Can you work these out from the model? Positions are in its coordinate system, mm. Face numbers are marked on the shaded views. A direction names the side the tool comes from. Coordinates: 2 decimals unless noted, no trailing zeros. Loops run counter-clockwise (first coordinate to the right, second up) from the corner with the lowest first, then second, coordinate; pieces in that order, holes last.
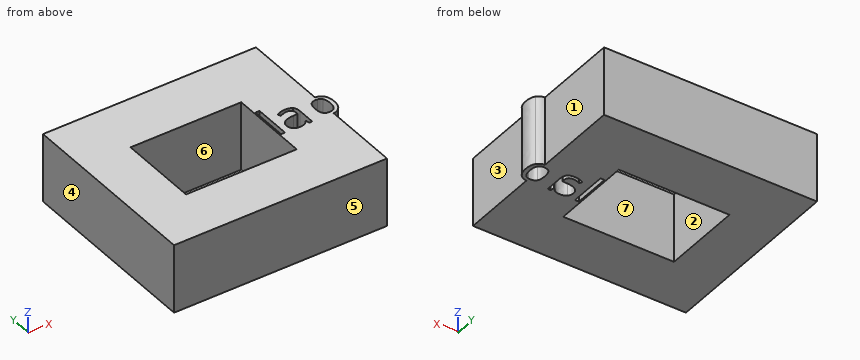
```python
from build123d import *

# Parameters (mm, degrees)
F0_W     = 1.4345356546
F0_H     = 13.4415161623
F1_DEPTH = 25


with BuildPart() as f1:
    # F0 (on Top) → F1 (new body)
    with BuildSketch(Plane.XY):
        Polygon((-19.7263322771, 14.6005926654), (-37.4334342778, 35.1035520434), (-37.4334342778, -33.8609479368), (-19.7263322771, -14.6005926654), align=None)
        Polygon((40.2292944491, 35.1035520434), (-37.4334342778, 35.1035520434), (-19.7263322771, 14.6005926654), (20.6582844257, 14.6005926654), align=None)
        with BuildLine():
            Line((40.2292944491, 4.0209012059), (40.2292944491, 35.1035520434))
            Line((40.2292944491, 35.1035520434), (20.6582844257, 14.6005926654))
            Line((20.6582844257, 14.6005926654), (20.6582844257, -14.6005926654))
            Line((20.6582844257, -14.6005926654), (40.2292944491, -33.8609479368))
            Line((40.2292944491, -33.8609479368), (40.2292944491, -5.7565652547))
            add(Edge.make_bspline(
                [(40.2292944491, -5.7565652547), (40.0783549242, -5.7658505375), (39.9216058908, -5.7658505375)],
                knots=[0.915231448, 0.915231448, 0.915231448, 1, 1, 1], degree=2))
            add(Edge.make_bspline(
                [(39.9216058908, -5.7658505375), (38.9956532043, -5.7658505375), (38.2313967333, -5.4244918605)],
                knots=[0, 0, 0, 1, 1, 1], degree=2))
            add(Edge.make_bspline(
                [(38.2313967333, -5.4244918605), (37.4671402622, -5.0831331836), (36.9502651805, -4.372775451)],
                knots=[0, 0, 0, 1, 1, 1], degree=2))
            Line((36.9502651805, -4.372775451), (36.8452317414, -4.372775451))
            Line((36.8452317414, -4.372775451), (36.5439516136, -5.5917161517))
            Line((36.5439516136, -5.5917161517), (35.5157295259, -5.5917161517))
            Line((35.5157295259, -5.5917161517), (35.5157295259, 7.8498000106))
            Line((35.5157295259, 7.8498000106), (36.9502651805, 7.8498000106))
            Line((36.9502651805, 7.8498000106), (36.9502651805, 4.5827072481))
            add(Edge.make_bspline(
                [(36.9502651805, 4.5827072481), (36.9502651805, 3.4853842137), (36.8811642337, 2.6147122846)],
                knots=[0, 0, 0, 1, 1, 1], degree=2))
            Line((36.8811642337, 2.6147122846), (36.9502651805, 2.6147122846))
            add(Edge.make_bspline(
                [(36.9502651805, 2.6147122846), (37.9508468894, 4.0298996741), (39.9216058908, 4.0298996741)],
                knots=[0, 0, 0, 1, 1, 1], degree=2))
            add(Edge.make_bspline(
                [(39.9216058908, 4.0298996741), (40.0783927276, 4.0298996741), (40.2292944491, 4.0209012059)],
                knots=[0, 0, 0, 0.0840353158, 0.0840353158, 0.0840353158], degree=2))
        make_face()
        with BuildLine():
            Line((32.5637370806, -5.5917161517), (31.4995825007, -5.5917161517))
            Line((31.4995825007, -5.5917161517), (31.2148866, -4.2428656711))
            Line((31.2148866, -4.2428656711), (31.1457856533, -4.2428656711))
            add(Edge.make_bspline(
                [(31.1457856533, -4.2428656711), (30.4381919585, -5.1328858652), (29.7347443206, -5.4493682014)],
                knots=[0, 0, 0, 1, 1, 1], degree=2))
            add(Edge.make_bspline(
                [(29.7347443206, -5.4493682014), (29.0312966827, -5.7658505375), (27.9754342163, -5.7658505375)],
                knots=[0, 0, 0, 1, 1, 1], degree=2))
            add(Edge.make_bspline(
                [(27.9754342163, -5.7658505375), (26.5685389404, -5.7658505375), (25.769731996, -5.0389085777)],
                knots=[0, 0, 0, 1, 1, 1], degree=2))
            add(Edge.make_bspline(
                [(25.769731996, -5.0389085777), (24.9709250515, -4.3119666178), (24.9709250515, -2.9741722887)],
                knots=[0, 0, 0, 1, 1, 1], degree=2))
            add(Edge.make_bspline(
                [(24.9709250515, -2.9741722887), (24.9709250515, -0.1078650174), (29.556463878, 0.0303368761)],
                knots=[0, 0, 0, 1, 1, 1], degree=2))
            Line((29.556463878, 0.0303368761), (31.1623698805, 0.0828535956))
            Line((31.1623698805, 0.0828535956), (31.1623698805, 0.6715936619))
            add(Edge.make_bspline(
                [(31.1623698805, 0.6715936619), (31.1623698805, 1.7855009236), (30.684191329, 2.3161961946)],
                knots=[0, 0, 0, 1, 1, 1], degree=2))
            add(Edge.make_bspline(
                [(30.684191329, 2.3161961946), (30.2060127774, 2.8468914657), (29.1501503111, 2.8468914657)],
                knots=[0, 0, 0, 1, 1, 1], degree=2))
            add(Edge.make_bspline(
                [(29.1501503111, 2.8468914657), (27.9671421027, 2.8468914657), (26.4745616528, 2.1227135437)],
                knots=[0, 0, 0, 1, 1, 1], degree=2))
            Line((26.4745616528, 2.1227135437), (26.0323155936, 3.2200365782))
            add(Edge.make_bspline(
                [(26.0323155936, 3.2200365782), (26.7316171747, 3.5987097664), (27.5649745926, 3.8143047202)],
                knots=[0, 0, 0, 1, 1, 1], degree=2))
            add(Edge.make_bspline(
                [(27.5649745926, 3.8143047202), (28.3983320104, 4.0298996741), (29.2385995229, 4.0298996741)],
                knots=[0, 0, 0, 1, 1, 1], degree=2))
            add(Edge.make_bspline(
                [(29.2385995229, 4.0298996741), (30.9301906994, 4.0298996741), (31.74696389, 3.2794633924)],
                knots=[0, 0, 0, 1, 1, 1], degree=2))
            add(Edge.make_bspline(
                [(31.74696389, 3.2794633924), (32.5637370806, 2.5290271106), (32.5637370806, 0.8706043886)],
                knots=[0, 0, 0, 1, 1, 1], degree=2))
            Line((32.5637370806, 0.8706043886), (32.5637370806, -5.5917161517))
        make_face(mode=Mode.SUBTRACT)
        with Locations((21.9208092619, 1.1290419294)):
            Rectangle(F0_W, F0_H, mode=Mode.SUBTRACT)
        Polygon((-19.7263322771, -14.6005926654), (-37.4334342778, -33.8609479368), (40.2292944491, -33.8609479368), (20.6582844257, -14.6005926654), align=None)
        with BuildLine():
            add(Edge.make_bspline(
                [(40.2292944491, 4.0209012059), (41.8740868362, 3.9228200715), (42.8196995976, 2.755678216)],
                knots=[0.0840353158, 0.0840353158, 0.0840353158, 1, 1, 1], degree=2))
            Line((40.2292944491, 4.0209012059), (40.2292944491, 2.7938202111))
            add(Edge.make_bspline(
                [(41.7168484874, 1.9237028171), (41.1987126844, 2.6484300811), (40.2292944491, 2.7938202111)],
                knots=[0, 0, 0, 0.7993864214, 0.7993864214, 0.7993864214], degree=2))
            add(Edge.make_bspline(
                [(42.365015368, -0.8320429394), (42.365015368, 1.0170983957), (41.7168484874, 1.9237028171)],
                knots=[0, 0, 0, 1, 1, 1], degree=2))
            add(Edge.make_bspline(
                [(41.7168484874, -3.6002268663), (42.365015368, -2.6369596686), (42.365015368, -0.8320429394)],
                knots=[0, 0, 0, 1, 1, 1], degree=2))
            add(Edge.make_bspline(
                [(40.2292944491, -4.528094354), (41.1929364436, -4.378833891), (41.7168484874, -3.6002268663)],
                knots=[0.1917019218, 0.1917019218, 0.1917019218, 1, 1, 1], degree=2))
            Line((40.2292944491, -4.528094354), (40.2292944491, -5.7565652547))
            add(Edge.make_bspline(
                [(42.811407484, -4.4736628332), (41.8589624891, -5.6563136569), (40.2292944491, -5.7565652547)],
                knots=[0, 0, 0, 0.915231448, 0.915231448, 0.915231448], degree=2))
            add(Edge.make_bspline(
                [(43.8520677421, -0.8486271666), (43.8520677421, -3.181475129), (42.811407484, -4.4736628332)],
                knots=[0, 0, 0, 1, 1, 1], degree=2))
            add(Edge.make_bspline(
                [(42.8196995976, 2.755678216), (43.8520677421, 1.4814567579), (43.8520677421, -0.8486271666)],
                knots=[0, 0, 0, 1, 1, 1], degree=2))
        make_face()
        with BuildLine():
            Line((40.2292944491, 2.7938202111), (40.2292944491, 4.0209012059))
            add(Edge.make_bspline(
                [(39.9216058908, 4.0298996741), (40.0783927276, 4.0298996741), (40.2292944491, 4.0209012059)],
                knots=[0, 0, 0, 0.0840353158, 0.0840353158, 0.0840353158], degree=2))
            add(Edge.make_bspline(
                [(36.9502651805, 2.6147122846), (37.9508468894, 4.0298996741), (39.9216058908, 4.0298996741)],
                knots=[0, 0, 0, 1, 1, 1], degree=2))
            Line((36.9502651805, 2.6147122846), (36.8811642337, 2.6147122846))
            add(Edge.make_bspline(
                [(36.9502651805, 4.5827072481), (36.9502651805, 3.4853842137), (36.8811642337, 2.6147122846)],
                knots=[0, 0, 0, 1, 1, 1], degree=2))
            Line((36.9502651805, 4.5827072481), (36.9502651805, 7.8498000106))
            Line((36.9502651805, 7.8498000106), (35.5157295259, 7.8498000106))
            Line((35.5157295259, 7.8498000106), (35.5157295259, -5.5917161517))
            Line((35.5157295259, -5.5917161517), (36.5439516136, -5.5917161517))
            Line((36.5439516136, -5.5917161517), (36.8452317414, -4.372775451))
            Line((36.8452317414, -4.372775451), (36.9502651805, -4.372775451))
            add(Edge.make_bspline(
                [(38.2313967333, -5.4244918605), (37.4671402622, -5.0831331836), (36.9502651805, -4.372775451)],
                knots=[0, 0, 0, 1, 1, 1], degree=2))
            add(Edge.make_bspline(
                [(39.9216058908, -5.7658505375), (38.9956532043, -5.7658505375), (38.2313967333, -5.4244918605)],
                knots=[0, 0, 0, 1, 1, 1], degree=2))
            add(Edge.make_bspline(
                [(40.2292944491, -5.7565652547), (40.0783549242, -5.7658505375), (39.9216058908, -5.7658505375)],
                knots=[0.915231448, 0.915231448, 0.915231448, 1, 1, 1], degree=2))
            Line((40.2292944491, -5.7565652547), (40.2292944491, -4.528094354))
            add(Edge.make_bspline(
                [(39.747471505, -4.563494064), (40.0007500207, -4.563494064), (40.2292944491, -4.528094354)],
                knots=[0, 0, 0, 0.1917019218, 0.1917019218, 0.1917019218], degree=2))
            add(Edge.make_bspline(
                [(37.6150162882, -3.7038782864), (38.279767396, -4.563494064), (39.747471505, -4.563494064)],
                knots=[0, 0, 0, 1, 1, 1], degree=2))
            add(Edge.make_bspline(
                [(36.9502651805, -0.8486271666), (36.9502651805, -2.8442625088), (37.6150162882, -3.7038782864)],
                knots=[0, 0, 0, 1, 1, 1], degree=2))
            add(Edge.make_bspline(
                [(37.598432061, 1.988657707), (36.9502651805, 1.1470081756), (36.9502651805, -0.8486271666)],
                knots=[0, 0, 0, 1, 1, 1], degree=2))
            add(Edge.make_bspline(
                [(39.7143030506, 2.8303072385), (38.2465989415, 2.8303072385), (37.598432061, 1.988657707)],
                knots=[0, 0, 0, 1, 1, 1], degree=2))
            add(Edge.make_bspline(
                [(40.2292944491, 2.7938202111), (39.9860097796, 2.8303072385), (39.7143030506, 2.8303072385)],
                knots=[0.7993864214, 0.7993864214, 0.7993864214, 1, 1, 1], degree=2))
        make_face()
    extrude(amount=F1_DEPTH)


solid = f1.part
```
(1) I want a section at C-C on z = 8.25. State how many separate pieces and enclosed holes the cut face has, then the cut area to 3 significant figures.
Check values:
separate pieces: 1
enclosed holes: 4
area: 4,100 mm2
(2) I want a section at B-B on y = -10.5. Write out the boundary of the cut face in (x, z).
Check values:
outline: (-37.43, 0) - (-19.73, 0) - (-19.73, 25) - (-37.43, 25) - close; (20.66, 0) - (40.23, 0) - (40.23, 25) - (20.66, 25) - close
(3) I want a section at A-A on x = -4. Write out the boundary of the cut face in (y, z).
Check values:
outline: (-33.86, 0) - (-14.6, 0) - (-14.6, 25) - (-33.86, 25) - close; (14.6, 0) - (35.1, 0) - (35.1, 25) - (14.6, 25) - close
(4) If we mould it in two halves opening along X, with no side actions, what happens to the marked faces 4, 5, 6 and 7? For each: released by +X, released by -X, zero draft, split by the parting line, or undercut.
Check values:
face 4: released by -X
face 5: zero draft
face 6: undercut
face 7: undercut
(5) I want a section at D-D on y = 27. Write out the boundary of the cut face in (x, z), then the cut area to 3 significant figures.
Check values:
outline: (-37.43, 0) - (40.23, 0) - (40.23, 25) - (-37.43, 25) - close
area: 1,940 mm2
(6) If I drill on probe 1 along X at (y, z) = (6, 10.25); probe 2 along X at (y, z) = (-7.5, 18.5); probe 3 along Y at (x, z) = (-5, 9), over which ranges is the centre line in solid material (lowest first)?
Check values:
probe 1: x = -37.43 to -19.73, 20.66 to 21.2, 22.64 to 40.23
probe 2: x = -37.43 to -19.73, 20.66 to 40.23
probe 3: y = -33.86 to -14.6, 14.6 to 35.1
(7) I'm going to push a flat-ended pin straight in: pin 1 (7.5 mm diameter, centred on y = -17, z = 15, fed in from +X). Where does the tip first touch, or does it pass through?
Check values:
pin 1: stops at x = 40.23
(8) Which directions (+Z, -Z, +X, -X, +Y, -Y) give clear straight access to the entire face, cutting with the end or side of a thin tool? Please do the marked faces 1, 2 and 3.
Check values:
face 1: +Z, -Z, +X, +Y
face 2: +Z, -Z
face 3: +Z, -Z, +X, -Y
